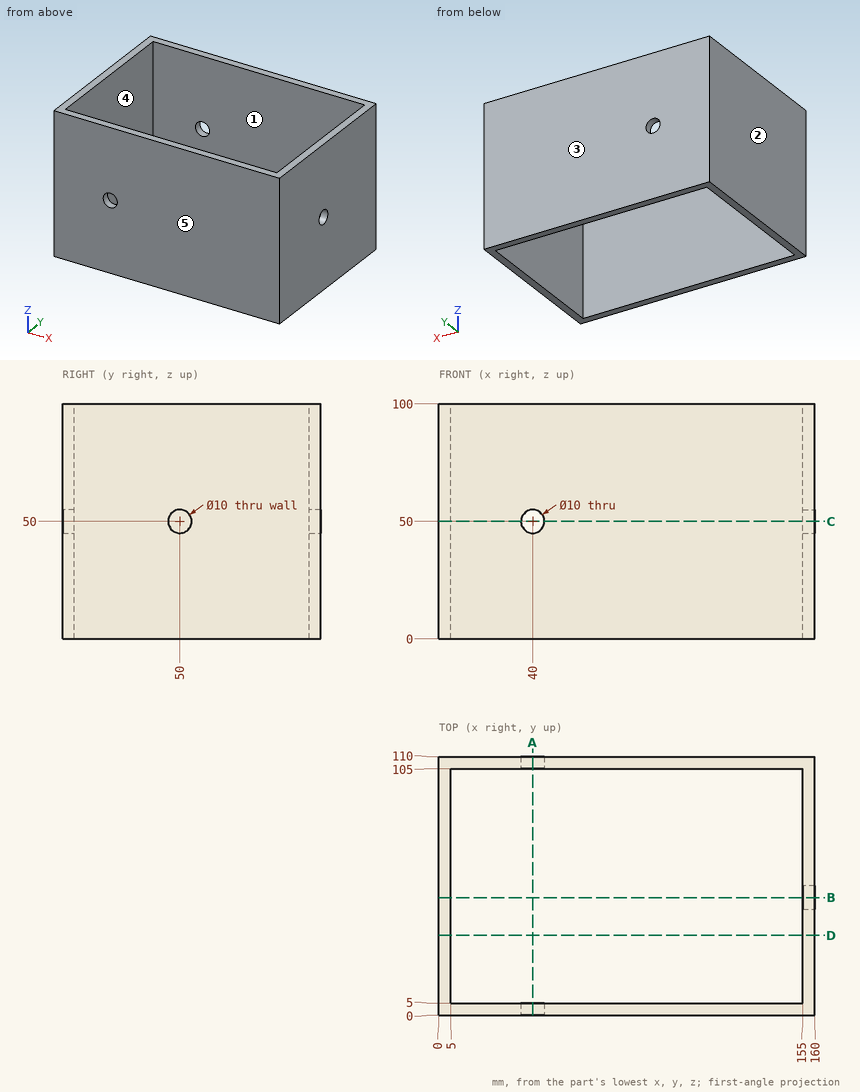
Study the drawing (mm; zero at the part's minimum x, y, z) and answer. A direction names the side the tool comes from. Give positions to 0.01 mm unless a question says otherwise; leave off trailing zeros. Loops run counter-clockwise (first coordinate to the right, second up) from the corner with the lowest first, then second, coordinate; pieces in that order, holes last. Notation, with made-up numbers: (37, 64.25) - (82, 64.25) arc R23 ccw to (82, 91.25) - close; hole circle Ø11 at (62.5, 87.5). An arc over 180 degrees is marked (long way). Use CSV: the item, a comma, the result in double quotes. Start each with the question number.
(1) Find section A-A, the plane x = 40. Determine the outline of the cut face in (y, z).
(2) Find section D-D, the plane y = 34. Determine the outline of the cut face in (x, z), plus the area to 3 significant figures.
(3) A tool of negligible diameter and unlimited length cuts with its end or side. For the marked faces 4 and 5, from which of +Z, -Z, +X, -X, +Y, -Y can it reach the whole face along a straight path? Write none if from no direction.
(4) Find the intervals of material crossed by L1, parallel to Y at x = 77, z = 71; L2, parallel to X at y = 34, z = 64.5; L3, parallel to X at y = 2.05, z = 50, in increasing order.
(5) This flat-tipped pin is pushed along its axis until it touches: pin 1 (8 mm diameter, centred on y = 50, z = 50, fed in from +X). Where does it stop, or does it pass through?
(6) Find section B-B, the plane y = 50. Determine the outline of the cut face in (x, z).
(7) Find section C-C, the plane z = 50. Determine the outline of the cut face in (x, y).
(8) Determine the mould class of the marked faces 1, 2 and 3 for opening direction X: released by +X, released by -X, zero draft, split by the parting line, or undercut.
Results found:
1,outline,"(0, 0) - (5, 0) - (5, 45) - (0, 45) - close; (0, 55) - (5, 55) - (5, 100) - (0, 100) - close; (105, 0) - (110, 0) - (110, 45) - (105, 45) - close; (105, 55) - (110, 55) - (110, 100) - (105, 100) - close"
2,outline,"(0, 0) - (5, 0) - (5, 100) - (0, 100) - close; (155, 0) - (160, 0) - (160, 100) - (155, 100) - close"
2,area,"1,000 mm^2"
3,face 4,"+Z, -Z"
3,face 5,"+Z, -Z, +X, -X, -Y"
4,L1,"0 to 5, 105 to 110"
4,L2,"0 to 5, 155 to 160"
4,L3,"0 to 35, 45 to 160"
5,pin 1,"x = 5"
6,outline,"(0, 0) - (5, 0) - (5, 100) - (0, 100) - close; (155, 0) - (160, 0) - (160, 45) - (155, 45) - close; (155, 55) - (160, 55) - (160, 100) - (155, 100) - close"
7,outline,"(0, 0) - (35, 0) - (35, 5) - (5, 5) - (5, 105) - (35, 105) - (35, 110) - (0, 110) - close; (45, 0) - (160, 0) - (160, 45) - (155, 45) - (155, 5) - (45, 5) - close; (45, 105) - (155, 105) - (155, 55) - (160, 55) - (160, 110) - (45, 110) - close"
8,face 1,"undercut"
8,face 2,"released by -X"
8,face 3,"zero draft"
